Model file for the job. Use its own axes, mm. Give positions to 0.01 mm unless a question says otherwise; leave off trailing zeros. Write each loop counter-clockwise with the first axis right and the second up, starting at its lowest first coordinate (ties: lowest second). Pieces come first, ordered by that corner, then holes. Notation, with made-up numbers: (55.25, 20) - (92.25, 20) arc R22 cw to (92.25, 27) - close; hole circle Ø6 at (75, -28). An arc over 180 degrees is marked (long way). Use CSV: the item, a comma, the result in double quotes.
from build123d import *

# Parameters (mm, degrees)
SKETCH_1_R          = 135.1
SKETCH_1_R_2        = 4
EXTRUDE_1_DEPTH     = 11.5
SKETCH_2_R          = 5
SKETCH_2_R_2        = 7
CUT_EXTRUDE_1_DEPTH = 23


with BuildPart() as part:
    # 草图1 → 凸台-拉伸1 (new, symmetric)
    with BuildSketch(Plane(origin=(0, 0, 0), x_dir=(1, 0, 0), z_dir=(0, 1, 0))):
        with BuildLine():
            Line((-180, 117.579760163), (-180, -117.579760163))
            ThreePointArc((-180, -117.579760163), (-140.706503078, -162.562849359), (-90.553851381, -195))
            Line((-90.553851381, -195), (90.553851381, -195))
            ThreePointArc((90.553851381, -195), (140.706503078, -162.562849359), (180, -117.579760163))
            Line((180, -117.579760163), (180, 117.579760163))
            ThreePointArc((180, 117.579760163), (140.706503078, 162.562849359), (90.553851381, 195))
            Line((90.553851381, 195), (-90.553851381, 195))
            ThreePointArc((-90.553851381, 195), (-140.706503078, 162.562849359), (-180, 117.579760163))
        make_face()
        with Locations(Location((0, 0, 0), (0, 0, 270))):
            Circle(SKETCH_1_R, mode=Mode.SUBTRACT)
        with Locations(Location((0, 145, 0), (0, 0, 270))):
            Circle(SKETCH_1_R_2, mode=Mode.SUBTRACT)
        with Locations(Location((72.5, 125.573683549, 0), (0, 0, 270))):
            Circle(SKETCH_1_R_2, mode=Mode.SUBTRACT)
        with Locations(Location((125.573683549, 72.5, 0), (0, 0, 270))):
            Circle(SKETCH_1_R_2, mode=Mode.SUBTRACT)
        with Locations(Location((145, 0, 0), (0, 0, 270))):
            Circle(SKETCH_1_R_2, mode=Mode.SUBTRACT)
        with Locations(Location((125.573683549, -72.5, 0), (0, 0, 270))):
            Circle(SKETCH_1_R_2, mode=Mode.SUBTRACT)
        with Locations(Location((72.5, -125.573683549, 0), (0, 0, 270))):
            Circle(SKETCH_1_R_2, mode=Mode.SUBTRACT)
        with Locations(Location((0, -145, 0), (0, 0, 270))):
            Circle(SKETCH_1_R_2, mode=Mode.SUBTRACT)
        with Locations(Location((-72.5, -125.573683549, 0), (0, 0, 270))):
            Circle(SKETCH_1_R_2, mode=Mode.SUBTRACT)
        with Locations(Location((-125.573683549, -72.5, 0), (0, 0, 270))):
            Circle(SKETCH_1_R_2, mode=Mode.SUBTRACT)
        with Locations(Location((-145, 0, 0), (0, 0, 270))):
            Circle(SKETCH_1_R_2, mode=Mode.SUBTRACT)
        with Locations(Location((-125.573683549, 72.5, 0), (0, 0, 270))):
            Circle(SKETCH_1_R_2, mode=Mode.SUBTRACT)
        with Locations(Location((-72.5, 125.573683549, 0), (0, 0, 270))):
            Circle(SKETCH_1_R_2, mode=Mode.SUBTRACT)
    extrude(amount=EXTRUDE_1_DEPTH, both=True)

    # 草图2 → 切除-拉伸1 (cut)
    with BuildSketch(Plane(origin=(0, 11.5, 0), x_dir=(1, 0, 0), z_dir=(0, 1, 0))):
        with Locations(Location((0, 175, 0), (0, 0, 270))):
            Circle(SKETCH_2_R)
        with Locations(Location((-30, 175, 0), (0, 0, 270))):
            Circle(SKETCH_2_R)
        with Locations(Location((-70, 175, 0), (0, 0, 270))):
            Circle(SKETCH_2_R_2)
        with Locations(Location((70, 175, 0), (0, 0, 90))):
            Circle(SKETCH_2_R_2)
        with Locations(Location((30, 175, 0), (0, 0, 90))):
            Circle(SKETCH_2_R)
        with Locations(Location((-70, -175, 0), (0, 0, 90))):
            Circle(SKETCH_2_R_2)
        with Locations(Location((-30, -175, 0), (0, 0, 90))):
            Circle(SKETCH_2_R)
        with Locations(Location((0, -175, 0), (0, 0, 90))):
            Circle(SKETCH_2_R)
        with Locations(Location((30, -175, 0), (0, 0, 270))):
            Circle(SKETCH_2_R)
        with Locations(Location((70, -175, 0), (0, 0, 270))):
            Circle(SKETCH_2_R_2)
        with Locations(Location((160, 85, 0), (0, 0, 270))):
            Circle(SKETCH_2_R_2)
        with Locations(Location((170, 30, 0), (0, 0, 270))):
            Circle(SKETCH_2_R)
        with Locations(Location((170, 0, 0), (0, 0, 270))):
            Circle(SKETCH_2_R)
        with Locations(Location((160, -85, 0), (0, 0, 90))):
            Circle(SKETCH_2_R_2)
        with Locations(Location((170, -30, 0), (0, 0, 90))):
            Circle(SKETCH_2_R)
        with Locations(Location((-170, -30, 0), (0, 0, 270))):
            Circle(SKETCH_2_R)
        with Locations(Location((-160, -85, 0), (0, 0, 270))):
            Circle(SKETCH_2_R_2)
        with Locations(Location((-170, 0, 0), (0, 0, 90))):
            Circle(SKETCH_2_R)
        with Locations(Location((-170, 30, 0), (0, 0, 90))):
            Circle(SKETCH_2_R)
        with Locations(Location((-160, 85, 0), (0, 0, 90))):
            Circle(SKETCH_2_R_2)
    extrude(amount=-CUT_EXTRUDE_1_DEPTH, mode=Mode.SUBTRACT)


solid = part.part
(1) Saw through at C-C, the plane x = -160. List the corners of the cut face in (y, z), then the cut area to 3 significant figures.
Checked values:
outline,"(-11.5, -143.61) - (11.5, -143.61) - (11.5, -92) - (-11.5, -92) - close; (-11.5, -78) - (11.5, -78) - (11.5, 78) - (-11.5, 78) - close; (-11.5, 92) - (11.5, 92) - (11.5, 143.61) - (-11.5, 143.61) - close"
area,"5,960 mm^2"
(2) Saw through at A-A, the plane x = 86. List the corners of the cut face in (y, z).
Checked values:
outline,"(-11.5, -195) - (11.5, -195) - (11.5, -104.19) - (-11.5, -104.19) - close; (-11.5, 104.19) - (11.5, 104.19) - (11.5, 195) - (-11.5, 195) - close"
(3) Saw through at D-D, the plane z = -175. List the corners of the cut face in (x, y), then the cut area to 3 significant figures.
Checked values:
outline,"(-124.9, -11.5) - (-77, -11.5) - (-77, 11.5) - (-124.9, 11.5) - close; (-63, -11.5) - (-35, -11.5) - (-35, 11.5) - (-63, 11.5) - close; (-25, -11.5) - (-5, -11.5) - (-5, 11.5) - (-25, 11.5) - close; (5, -11.5) - (25, -11.5) - (25, 11.5) - (5, 11.5) - close; (35, -11.5) - (63, -11.5) - (63, 11.5) - (35, 11.5) - close; (77, -11.5) - (124.9, -11.5) - (124.9, 11.5) - (77, 11.5) - close"
area,"4,410 mm^2"
(4) Flat gauge pins, fed straight in: P1, Ø6, axis at x = -109, y = 0, coming from the -Z side; P2, Ø6, axis at x = -104, y = 2.5, coming from the -Z side; P3, Ø4, axis at x = -142, y = 9, coming from the -Z side. Where does each tip first touch, or does it go through?
Checked values:
P1,"stops at z = -187.05"
P2,"stops at z = -189.8"
P3,"stops at z = -163.17"
(5) Wall check: probe 1 along X at (y, z) = (5.5, 0); probe 2 along Z at (x, y) = (28.5, 2.5); probe 3 along Z at (x, y) = (72, 10). Give the ranges that are in metal, low to high. Write a range as [from, to].
Checked values:
probe 1,"x = [-180, -175], [-165, -149], [-141, -135.1], [135.1, 141], [149, 165], [175, 180]"
probe 2,"z = [-195, -179.77], [-170.23, -132.06], [132.06, 170.23], [179.77, 195]"
probe 3,"z = [-195, -181.71], [-168.29, -129.54], [-121.61, -114.32], [114.32, 121.61], [129.54, 168.29], [181.71, 195]"
(6) Pull direction Z, two halves, no side cores. Call faces 1 (the face through (37, 11.5, -133)), 2 (the face through (141.34, 0.16, -162.01)), 3 (the face through (-165.043, 0.161, 29.349)): released by +Z, released by -Z, zero draft, split by the parting line, or undercut.
Checked values:
face 1,"zero draft"
face 2,"released by -Z"
face 3,"undercut"
(7) Saw through at B-B, the plane z = 30.5. List the corners of the cut face in (x, y), then the cut area to 3 significant figures.
Checked values:
outline,"(-180, -11.5) - (-174.97, -11.5) - (-174.97, 11.5) - (-180, 11.5) - close; (-165.03, -11.5) - (-131.61, -11.5) - (-131.61, 11.5) - (-165.03, 11.5) - close; (131.61, -11.5) - (165.03, -11.5) - (165.03, 11.5) - (131.61, 11.5) - close; (174.97, -11.5) - (180, -11.5) - (180, 11.5) - (174.97, 11.5) - close"
area,"1,770 mm^2"
